from build123d import *

# Parameters (mm, degrees)
F1_DEPTH     = 6
F3_DEPTH     = 5.2
F4_T1_DEPTH  = 13.92
F4_T3_DEPTH  = 5.5
F4_T6_ANGLE  = 90
F4_T8_ANGLE  = 90
F4_T10_ANGLE = 90
F4_T12_ANGLE = 90
F4_T14_ANGLE = 90
F4_T16_ANGLE = 90
F4_T18_ANGLE = 90
F4_T20_ANGLE = 90


# Not quite as in the source:
# - a fillet or chamfer that OpenCascade refuses, or shapes differently, is made with other operations: its cross-section is extruded or revolved along the edge and cut away or added


with BuildPart() as f1:
    # F0 (on Top) → F1 (new body)
    with BuildSketch(Plane.XY):
        with BuildLine():
            Line((6.96, 5.75), (-6.96, 5.75))
            ThreePointArc((-6.96, 5.75), (-9.0813203436, 4.8713203436), (-9.96, 2.75))
            Line((-9.96, 2.75), (-9.96, -2.75))
            ThreePointArc((-9.96, -2.75), (-9.0813203436, -4.8713203436), (-6.96, -5.75))
            Line((-6.96, -5.75), (6.96, -5.75))
            ThreePointArc((6.96, -5.75), (9.0813203436, -4.8713203436), (9.96, -2.75))
            Line((9.96, -2.75), (9.96, 2.75))
            ThreePointArc((9.96, 2.75), (9.0813203436, 4.8713203436), (6.96, 5.75))
        make_face()
    extrude(amount=F1_DEPTH)

    # F2 (on face) → F3 (cut)
    with BuildSketch(Plane.XY.offset(6)):
        Polygon((2.95, 5.1095498823), (-2.95, 5.1095498823), (-5.9, 0), (-2.95, -5.1095498823), (2.95, -5.1095498823), (5.9, 0), align=None)
    extrude(amount=-F3_DEPTH, mode=Mode.SUBTRACT)

    # F4: chamfer of 1 on 2 edges, made by hand

    # F4_s2 → F4_t1 (cut)
    with BuildSketch(Plane.YZ.offset(-6.96)):
        Polygon((5.75, 5), (4.75, 6), (5.75, 6), align=None)
        Polygon((5.75, 1), (4.75, 0), (5.75, 0), align=None)
        Polygon((-4.75, 0), (-5.75, 1), (-5.75, 0), align=None)
        Polygon((-4.75, 6), (-5.75, 5), (-5.75, 6), align=None)
    extrude(amount=F4_T1_DEPTH, mode=Mode.SUBTRACT)

    # F4_s4 → F4_t3 (cut)
    with BuildSketch(Plane.XZ.offset(-2.75)):
        Polygon((-8.96, 0), (-9.96, 1), (-9.96, 0), align=None)
        Polygon((8.96, 0), (9.96, 1), (9.96, 0), align=None)
        Polygon((-8.96, 6), (-9.96, 5), (-9.96, 6), align=None)
        Polygon((8.96, 6), (9.96, 5), (9.96, 6), align=None)
    extrude(amount=F4_T3_DEPTH, mode=Mode.SUBTRACT)

    # F4_s5 → F4_t6 (revolve, cut)
    with BuildSketch(Plane.XZ.offset(-2.75)):
        Polygon((9.96, 1), (8.96, 0), (9.96, 0), align=None)
    revolve(axis=Axis((6.96, 2.75, 0), (0, 0, 1)), revolution_arc=F4_T6_ANGLE, mode=Mode.SUBTRACT)

    # F4_s7 → F4_t8 (revolve, cut)
    with BuildSketch(Plane.YZ.offset(-6.96)):
        Polygon((5.75, 1), (4.75, 0), (5.75, 0), align=None)
    revolve(axis=Axis((-6.96, 2.75, 0), (0, 0, 1)), revolution_arc=F4_T8_ANGLE, mode=Mode.SUBTRACT)

    # F4_s9 → F4_t10 (revolve, cut)
    with BuildSketch(Plane.XZ.offset(2.75)):
        Polygon((-8.96, 0), (-9.96, 1), (-9.96, 0), align=None)
    revolve(axis=Axis((-6.96, -2.75, 0), (0, 0, 1)), revolution_arc=F4_T10_ANGLE, mode=Mode.SUBTRACT)

    # F4_s11 → F4_t12 (revolve, cut)
    with BuildSketch(Plane.YZ.offset(6.96)):
        Polygon((-4.75, 0), (-5.75, 1), (-5.75, 0), align=None)
    revolve(axis=Axis((6.96, -2.75, 0), (0, 0, 1)), revolution_arc=F4_T12_ANGLE, mode=Mode.SUBTRACT)

    # F4_s13 → F4_t14 (revolve, cut)
    with BuildSketch(Plane.XZ.offset(-2.75)):
        Polygon((9.96, 5), (8.96, 6), (9.96, 6), align=None)
    revolve(axis=Axis((6.96, 2.75, 6), (0, 0, 1)), revolution_arc=F4_T14_ANGLE, mode=Mode.SUBTRACT)

    # F4_s15 → F4_t16 (revolve, cut)
    with BuildSketch(Plane.YZ.offset(-6.96)):
        Polygon((5.75, 5), (4.75, 6), (5.75, 6), align=None)
    revolve(axis=Axis((-6.96, 2.75, 6), (0, 0, 1)), revolution_arc=F4_T16_ANGLE, mode=Mode.SUBTRACT)

    # F4_s17 → F4_t18 (revolve, cut)
    with BuildSketch(Plane.XZ.offset(2.75)):
        Polygon((-8.96, 6), (-9.96, 5), (-9.96, 6), align=None)
    revolve(axis=Axis((-6.96, -2.75, 6), (0, 0, 1)), revolution_arc=F4_T18_ANGLE, mode=Mode.SUBTRACT)

    # F4_s19 → F4_t20 (revolve, cut)
    with BuildSketch(Plane.YZ.offset(6.96)):
        Polygon((-4.75, 6), (-5.75, 5), (-5.75, 6), align=None)
    revolve(axis=Axis((6.96, -2.75, 6), (0, 0, 1)), revolution_arc=F4_T20_ANGLE, mode=Mode.SUBTRACT)


solid = f1.part
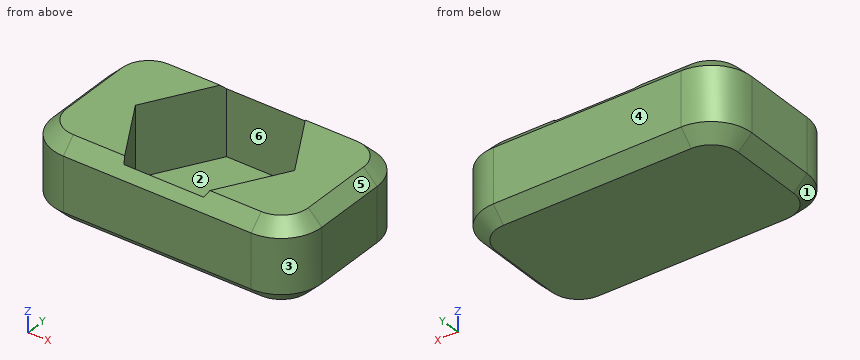
Model file for the job. Use its own axes, mm. Face numbers are marked on the shaded views. A direction names the side the tool comes from. Round coordinates to 2 decimals unless told otherwise and drop trailing zeros. Loops run counter-clockwise (first coordinate to the right, second up) from the corner with the lowest first, then second, coordinate; pieces in that order, holes last. Notation, with made-up numbers: (29, 40.25) - (42, 40.25) arc R8 cw to (42, 47.25) - close; hole circle Ø1 at (-24, 45). An arc over 180 degrees is marked (long way). Write each question's results on one line, items separated by ' | '.
(1) Mould opens along X. For the marked faces 1, 2, 3 and 4 say: released by +X, released by -X, zero draft, split by the parting line, or undercut.
Answer below:
face 1: released by -X | face 2: undercut | face 3: released by +X | face 4: zero draft
(2) Saw through at A-A, the plane z = 3.3. List the corners of the cut face in (x, y), then the cut area to 3 significant figures.
Answer below:
outline: (-9.96, -2.75) arc R3 ccw to (-6.96, -5.75) - (6.96, -5.75) arc R3 ccw to (9.96, -2.75) - (9.96, 2.75) arc R3 ccw to (6.96, 5.75) - (-6.96, 5.75) arc R3 ccw to (-9.96, 2.75) - close; hole (-5.9, 0) - (-2.95, -5.11) - (2.95, -5.11) - (5.9, 0) - (2.95, 5.11) - (-2.95, 5.11) - close | area: 131 mm^2
(3) Saw through at B-B, the plane x = 2.5. List the corners of the cut face in (y, z).
Answer below:
outline: (-5.75, 1) - (-4.75, 0) - (4.75, 0) - (5.75, 1) - (5.75, 5) - (5.11, 5.64) - (5.11, 0.8) - (-5.11, 0.8) - (-5.11, 5.64) - (-5.75, 5) - close
(4) Wall check: L1, parallel to X at y = 2, z = 2.45; L2, parallel to Y at x = -2.75, z = 1.65; L3, parallel to Z at x = 4.25, y = 2.5. Give the ranges that are in metal, low to high.
Answer below:
L1: x = -9.96 to -4.75, 4.75 to 9.96 | L2: y = -5.75 to -5.11, 5.11 to 5.75 | L3: z = 0 to 0.8
(5) Saw through at D-D, the plane z = 5.25. List the corners of the cut face in (x, y), then the cut area to 3 significant figures.
Answer below:
outline: (-9.71, -2.75) arc R2.75 ccw to (-6.96, -5.5) - (6.96, -5.5) arc R2.75 ccw to (9.71, -2.75) - (9.71, 2.75) arc R2.75 ccw to (6.96, 5.5) - (-6.96, 5.5) arc R2.75 ccw to (-9.71, 2.75) - close; hole (-5.9, 0) - (-2.95, -5.11) - (2.95, -5.11) - (5.9, 0) - (2.95, 5.11) - (-2.95, 5.11) - close | area: 117 mm^2
(6) Saw through at C-C, the plane y = 2. List the corners of the cut face in (x, z).
Answer below:
outline: (-9.96, 1) - (-8.96, 0) - (8.96, 0) - (9.96, 1) - (9.96, 5) - (8.96, 6) - (4.75, 6) - (4.75, 0.8) - (-4.75, 0.8) - (-4.75, 6) - (-8.96, 6) - (-9.96, 5) - close
(7) Pin check, flat tip, straight feed: pin 1 (1 mm diameter, centred on y = -3.5, z = 0.5, fed in from -X). Stop position of the tip, or through.
Answer below:
pin 1: stops at x = -9.88
(8) 3-axis set-ups, long thin cutter, end or side, ignore diameter. For the marked faces 5 and 6: which of +Z, -Z, +X, -X, +Y, -Y reach the whole face in a straight line?
Answer below:
face 5: +Z, +X, +Y, -Y | face 6: +Z
